Design review of the part built by this model. Coordinates are the model's own, in mm. A direction names the side the tool comes from. Coordinates: 2 decimals unless noted, no trailing zeros. One line per item, written item: value.
from build123d import *

# Parameters (mm, degrees)
F0_R     = 11.15
F1_DEPTH = 7
F2_R     = 31.4472101729
F3_R     = 2.5


with BuildPart() as f1:
    # F0 (on Top) → F1 (new body)
    with BuildSketch(Plane.XY):
        with BuildLine():
            Line((20.1671623726, 11.6435166246), (12.9445725954, 38.4833765179))
            ThreePointArc((12.9445725954, 38.4833765179), (0, 48.4050688787), (-12.9445725954, 38.4833765179))
            Line((-12.9445725954, 38.4833765179), (-20.1671623726, 11.6435166246))
            Line((-20.1671623726, 11.6435166246), (-39.7998679856, -8.0313595503))
            ThreePointArc((-39.7998679856, -8.0313595503), (-41.9200193209, -24.2025344393), (-26.8552953903, -30.4520169677))
            Line((-26.8552953903, -30.4520169677), (0, -23.2870332492))
            Line((0, -23.2870332492), (26.8552953903, -30.4520169677))
            ThreePointArc((26.8552953903, -30.4520169677), (41.9200193209, -24.2025344393), (39.7998679856, -8.0313595503))
            Line((39.7998679856, -8.0313595503), (20.1671623726, 11.6435166246))
        make_face()
        Polygon((-35.9108891325, -14.2668384925), (-30.3108891325, -11.0336769851), (-24.7108891325, -14.2668384925), (-24.7108891325, -20.7331615075), (-30.3108891325, -23.9663230149), (-35.9108891325, -20.7331615075), align=None, mode=Mode.SUBTRACT)
        Polygon((-16.1608891325, -23.8797204745), (-21.7108891325, -20.6754264805), (-21.7108891325, -14.2668384925), (-16.1608891325, -11.0625444985), (-10.6108891325, -14.2668384925), (-10.6108891325, -20.6754264805), align=None, mode=Mode.SUBTRACT)
        Polygon((-23.2108891325, 1.1484136948), (-17.6608891325, -2.0558802992), (-17.6608891325, -8.4644682872), (-23.2108891325, -11.6687622812), (-28.7608891325, -8.4644682872), (-28.7608891325, -2.0558802992), align=None, mode=Mode.SUBTRACT)
        Polygon((10.6108891325, -20.6754264805), (10.6108891325, -14.2668384925), (16.1608891325, -11.0625444985), (21.7108891325, -14.2668384925), (21.7108891325, -20.6754264805), (16.1608891325, -23.8797204745), align=None, mode=Mode.SUBTRACT)
        Polygon((30.3108891325, -23.9663230149), (24.7108891325, -20.7331615075), (24.7108891325, -14.2668384925), (30.3108891325, -11.0336769851), (35.9108891325, -14.2668384925), (35.9108891325, -20.7331615075), align=None, mode=Mode.SUBTRACT)
        Circle(F0_R, mode=Mode.SUBTRACT)
        Polygon((28.7608891325, -2.0558802992), (28.7608891325, -8.4644682872), (23.2108891325, -11.6687622812), (17.6608891325, -8.4644682872), (17.6608891325, -2.0558802992), (23.2108891325, 1.1484136948), align=None, mode=Mode.SUBTRACT)
        Polygon((-7.05, 29.1398947677), (-1.5, 25.9356007737), (-1.5, 21.6791189615), (-1.5, 19.5270127857), (-7.05, 16.3227187917), (-11.8772290867, 19.1097208044), (-12.6, 19.5270127857), (-12.6, 25.9356007737), (-10.7562631022, 27.000082768), align=None, mode=Mode.SUBTRACT)
        Polygon((10.7562631022, 27.000082768), (12.6, 25.9356007737), (12.6, 19.5270127857), (11.8772290867, 19.1097208044), (7.05, 16.3227187917), (1.5, 19.5270127857), (1.5, 21.6791189615), (1.5, 25.9356007737), (7.05, 29.1398947677), align=None, mode=Mode.SUBTRACT)
        Polygon((0, 41.4663230149), (5.6, 38.2331615075), (5.6, 31.7668384925), (0, 28.5336769851), (-5.6, 31.7668384925), (-5.6, 38.2331615075), align=None, mode=Mode.SUBTRACT)
    extrude(amount=F1_DEPTH)

    # F2
    f2_edges = [f1.edges().sort_by_distance(p)[0] for p in [
        (20.167162, 11.643517, 3.5),
        (-20.167162, 11.643517, 3.5),
        (0, -23.287033, 3.5),
    ]]
    fillet(f2_edges, radius=F2_R)

    # F3
    f3_edges = [f1.edges().sort_by_distance(p)[0] for p in [
        (-32.946681, -1.163452, 7),
        (-21.11979, 12.193517, 0),
    ]]
    fillet(f3_edges, radius=F3_R)


solid = f1.part
1. For faces 1 (the face through (-17.543, -27.19, 6.287)), 2 (the face through (-20.397, -10.044, 3.451)), 3 (the face through (-17.543, -27.19, 0.713)), 4 (the face through (-21.063, 12.293, 3.514)), list the 3-axis set-ups (+Z, -Z, +X, -X, +Y, -Y) from which the entire face can be reached by the end or side of a thin tool; tool diameter is ignored.
Answer block:
face 1: +Z, -Y
face 2: +Z, -Z
face 3: -Z, -Y
face 4: +Z, -Z, -X, +Y
2. Consider section A-A, the plane z = 1. Give the number of separate pieces and of enclosed holes in the cut face, then the cut area to 3 significant figures.
Answer block:
separate pieces: 1
enclosed holes: 10
area: 2,470 mm^2
3. Wall thickness on line 1 along Y through (x, z) = (20.5, 2); line 2 along Y through (x, z) = (28, 4.5); line 3 along X through (y, z) = (18, 3.25): over which ranges is each line inside the solid? List them lowest first.
Answer block:
line 1: y = -28.7 to -21.37, -13.57 to -10.1, -0.42 to 13.21
line 2: y = -30.7 to -22.63, -12.37 to -8.9, -1.62 to 3.79
line 3: x = -18.51 to -9.96, -4.14 to 4.14, 9.96 to 18.51
4. Insertion check: pin 1 Ø4 at (x, z) = (-33.5, 4) entering from -Y; pin 2 Ø3 at (y, z) = (24, 4.5) entering from +X; pin 3 Ø1.9 at (y, z) = (-19, 4) entering from -X; pin 4 Ø10 at (x, y) = (5.5, -21) entering from -Z. Each pin has a flat end and moves straight along its axis. Give the tip position at first contact, or say it passes through.
Answer block:
pin 1: stops at y = -30.85
pin 2: stops at x = 17.25
pin 3: stops at x = -43.7
pin 4: stops at z = 0
5. Mouldability with a two-part tool opening along Y and no side actions: class faces 5 (the face through (33.2, -22.3, 3.5)), 6 (the face through (17.81, -27.26, 0.71)), 7 (the face through (14.7, 29.05, 6.29)) as released by +Y, released by -Y, zero draft, split by the parting line, or undercut.
Answer block:
face 5: undercut
face 6: released by -Y
face 7: released by +Y
